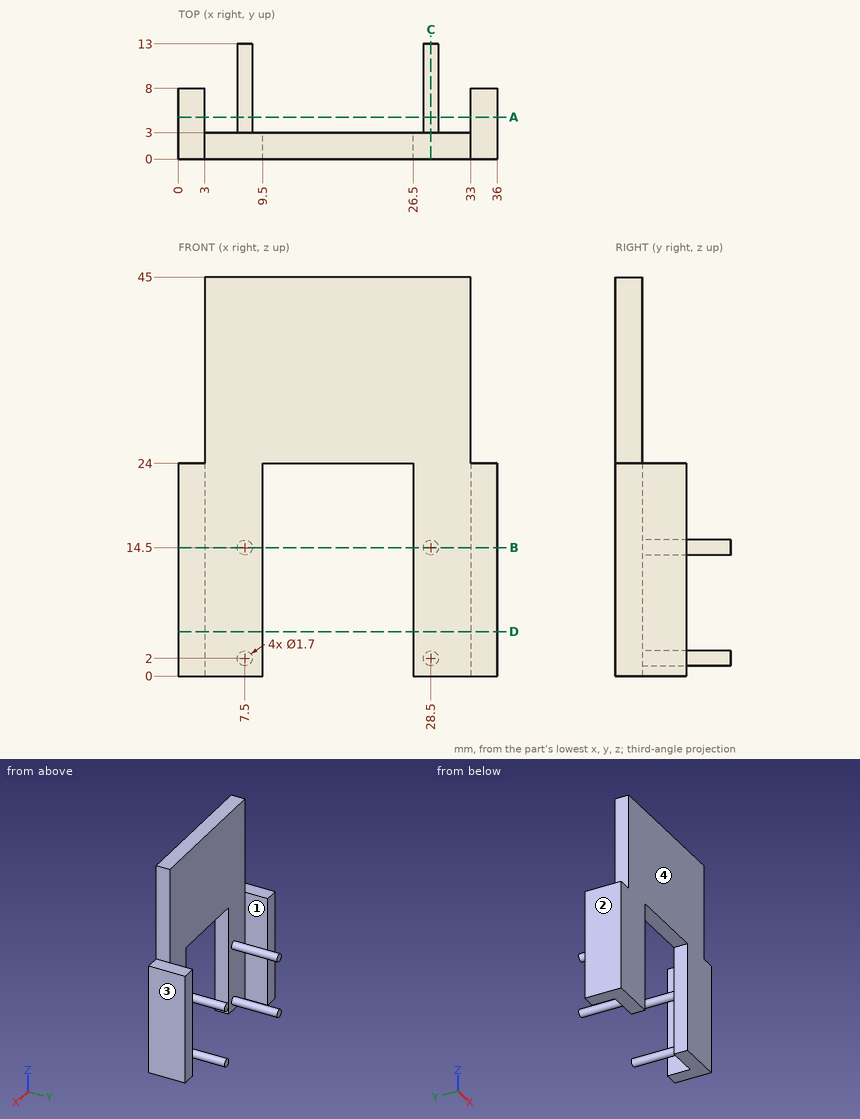
Geometry check sheet. Reference: drawing and pictorial views, mm from the part's lowest x, y, z. Coordinates: 2 decimals unless noted, no trailing zeros. Order: outer loops, then holes, each group sorted by start corner. A loop starts at its lowest first (then second) coordinate and runs counter-clockwise, first axis right, second up. Notation, with made-up numbers: M 86.25,60.25 L 107.25,60.25 A16 ccw 107.25,86.25 Z; hole C -27.5,77 d2. An arc over 180 degrees is marked long. Return JSON: item names as keys, results as strings.
1) Cross-section at B-B, the plane z = 14.5. Record the boundary of the cut face in (x, y), and give its area (3 significant figures).
Answer list:
{"outline": "M 0,0 L 9.5,0 L 9.5,3 L 8.35,3 L 8.35,13 L 6.65,13 L 6.65,3 L 3,3 L 3,8 L 0,8 Z; M 26.5,0 L 36,0 L 36,8 L 33,8 L 33,3 L 29.35,3 L 29.35,13 L 27.65,13 L 27.65,3 L 26.5,3 Z", "area": "121 mm2"}
2) Cross-section at A-A, the plane y = 4.75. Record the boundary of the cut face in (x, z), and give its area (3 significant figures).
Answer list:
{"outline": "M 0,0 L 3,0 L 3,24 L 0,24 Z; C 7.5,2 d1.7; C 7.5,14.5 d1.7; C 28.5,2 d1.7; C 28.5,14.5 d1.7; M 33,0 L 36,0 L 36,24 L 33,24 Z", "area": "153 mm2"}
3) Cross-section at C-C, the plane x = 28.5. Record the boundary of the cut face in (y, z), and give its area (3 significant figures).
Answer list:
{"outline": "M 0,0 L 3,0 L 3,1.15 L 13,1.15 L 13,2.85 L 3,2.85 L 3,13.65 L 13,13.65 L 13,15.35 L 3,15.35 L 3,45 L 0,45 Z", "area": "169 mm2"}
4) Thickness scan on L1, parallel to X at y = 2, z = 22.5; L2, parallel to Y at x = 25.5, z = 38; L3, parallel to X at y = 2.75, z = 29.5. Record the ranges inside material, lowest first. Write a range as [from, to].
Answer list:
{"L1": "[0, 9.5], [26.5, 36]", "L2": "[0, 3]", "L3": "[3, 33]"}
5) Gauge pin test, flat ends, axial feed: pin 1 (3.5 mm diameter, centred on x = 35, y = 6, fed in from +Z); pin 2 (8 mm diameter, centred on x = 14.5, z = 37, fed in from +Y); pin 3 (1.5 mm diameter, centred on y = 1, z = 39, fed in from -X). Record the tip position at first contact, or that the pin passes through.
Answer list:
{"pin 1": "z = 24", "pin 2": "y = 3", "pin 3": "x = 3"}
6) Release check for a two-part mould opening along X. For the marked faces 1, 2, 3 and 4 record: +X half, -X half, draft (parallel to the pull), parting line (faces both ways), or undercut.
Answer list:
{"face 1": "undercut", "face 2": "-X half", "face 3": "+X half", "face 4": "draft"}
7) Cross-section at D-D, the plane z = 5. Record the boundary of the cut face in (x, y).
Answer list:
{"outline": "M 0,0 L 9.5,0 L 9.5,3 L 3,3 L 3,8 L 0,8 Z; M 26.5,0 L 36,0 L 36,8 L 33,8 L 33,3 L 26.5,3 Z"}
